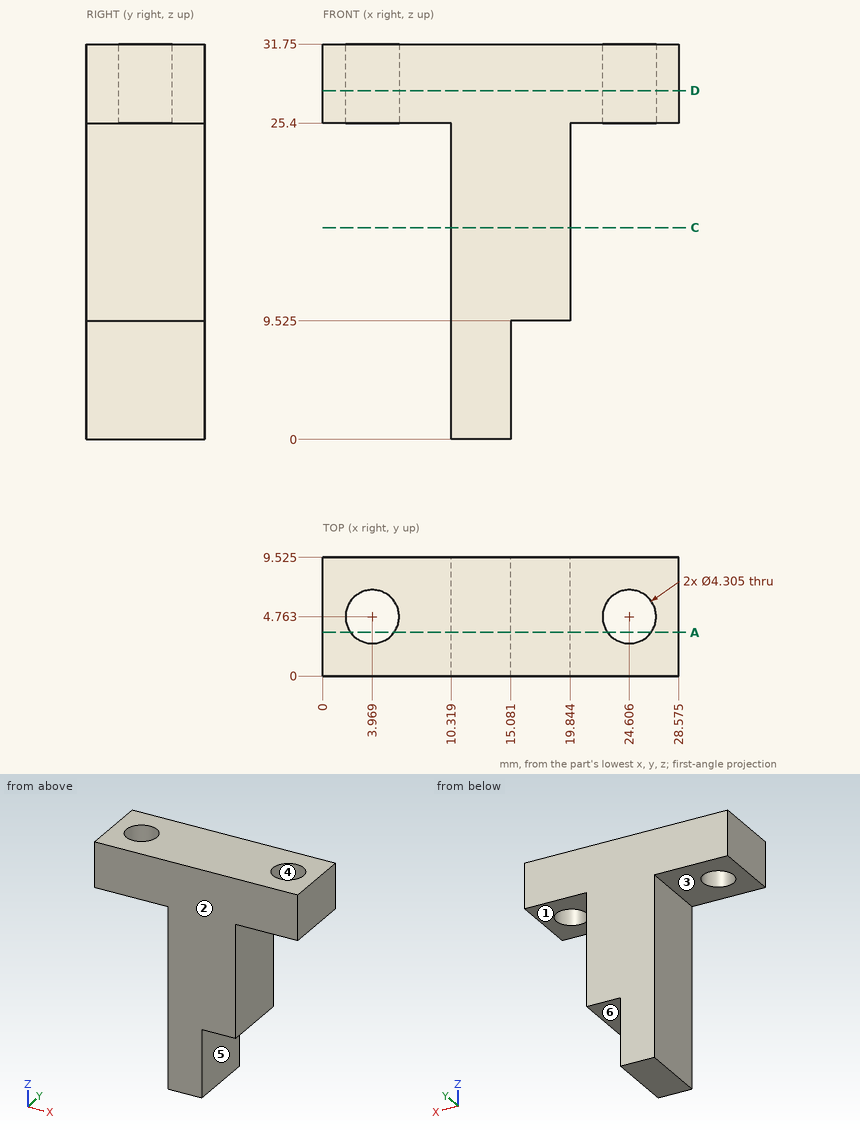
Input: dimensioned drawing with shaded views. Units: mm. Origin: part minimum x, y, z. A direction names the side the tool comes from. Round coordinates to 2 decimals unless told otherwise and drop trailing zeros. Loops run counter-clockwise (first coordinate to the right, second up) from the corner with the lowest first, then second, coordinate; pieces in that order, holes last. Notation, with made-up numbers: M -22.5,41.5 L 28.5,41.5 A24 cw 28.5,69.5 Z; hole C -19,-11 d8. An arc over 180 degrees is marked long. Return JSON: item names as keys, results as strings. Group by question number.
1. Section query C-C on z = 17. Output: boundary loops of the cut face in (x, y) (1 decimal).
2. Reachability of the marked faces 1, 2 and 3 from +Z, -Z, +X, -X, +Y, -Y: full face, straight path, thin tool, end or side. Return the list, or none.
3. Pin query (flat end, axial travel): pin 1 (3 mm diameter, centred on y = 7, z = 6, fed in from +X); pin 2 (1.5 mm diameter, centred on x = 13.5, y = 6.5, fed in from -Z); pin 3 (3 mm diameter, centred on y = 6.5, z = 15, fed in from -X); pin 4 (1.4 mm diameter, centred on x = 18, y = 5, fed in from -Z) (1 decimal). Return the tip coordinate at first contact, or that it passes through.
4. Section query A-A on y = 3.5. State how many separate pieces and enclosed holes the cut face has, and give its area (3 significant figures).
5. Material intervals for line 1 along X through (y, z) = (3.75, 30.5) (1 decimal); line 2 along X through (y, z) = (8.75, 3.5); line 3 along Z through (x, y) = (21.25, 7.5), sorted ascending. Write a range as from..to.
6. Section query D-D on z = 28. Output: boundary loops of the cut face in (x, y) (1 decimal), and give its area (3 significant figures).
7. Mould query, pull axis X, two halves, no side actions, for the marked faces 4, 5 and 6. Classes: released by +X, released by -X, zero draft, split by the parting line, or undercut.
Checks:
{
 "1": {"outline": "M 10.3,0 L 19.8,0 L 19.8,9.5 L 10.3,9.5 Z"},
 "2": {"face 1": "-Z, +X, +Y, -Y", "face 2": "+Z, -Z, +X, -X, -Y", "face 3": "-Z, -X, +Y, -Y"},
 "3": {"pin 1": "stops at x = 15.08", "pin 2": "stops at z = 0", "pin 3": "stops at x = 10.32", "pin 4": "stops at z = 9.5"},
 "4": {"separate pieces": "3", "enclosed holes": "0", "area": "334 mm²"},
 "5": {"line 1": "x = 0..2.1, 5.9..22.7, 26.5..28.6", "line 2": "x = 10.32..15.08", "line 3": "z = 25.4..31.75"},
 "6": {"outline": "M 0,0 L 28.6,0 L 28.6,9.5 L 0,9.5 Z; hole C 4,4.8 d4.3; hole C 24.6,4.8 d4.3", "area": "243 mm²"},
 "7": {"face 4": "undercut", "face 5": "released by +X", "face 6": "zero draft"}
}
